The model under review builds one solid part; all positions refer to its coordinate system, in mm. Face numbers are marked on the shaded views. A direction names the side the tool comes from. Round coordinates to 2 decimals unless told otherwise and drop trailing zeros. Loops run counter-clockwise (first coordinate to the right, second up) from the corner with the lowest first, then second, coordinate; pieces in that order, holes last. Notation, with made-up numbers: (-25, 72.5) -> (-10, 72.5) arc R21 cw to (-10, 84.5) -> close; hole circle Ø5 at (80, 50.25). An arc over 180 degrees is marked (long way). Use a Markdown table: item, result. Add a question column.
1) Wall thickness on probe 1 along Z at (x, y) = (3, -4); probe 2 along Z at (x, y) = (7, -16.5); probe 3 along X at (y, z) = (-17.75, -14.75): over which ranges is each line inside the solid? List them lowest first.
2) Mouldability with a two-part tool opening along X and no side actions: class the marked faces 1, 2, 3 and 4 as released by +X, released by -X, zero draft, split by the parting line, or undercut.
3) Consider section A-A on y = -3.75. Give the boundary of the cut face in (x, z), plus the area to 3 significant figures.
4) Insertion check: pin 1 (2.5 mm diameter, centred on x = 11, z = -3, fed in from +Y). The pin has a flat end and moves straight along its axis. Give the tip position at first contact, or say it passes through.
5) For the marked faces 5, 6 and 7, list the 3-axis set-ups (+Z, -Z, +X, -X, +Y, -Y) from which the entire face can be reached by the end or side of a thin tool; tool diameter is ignored.
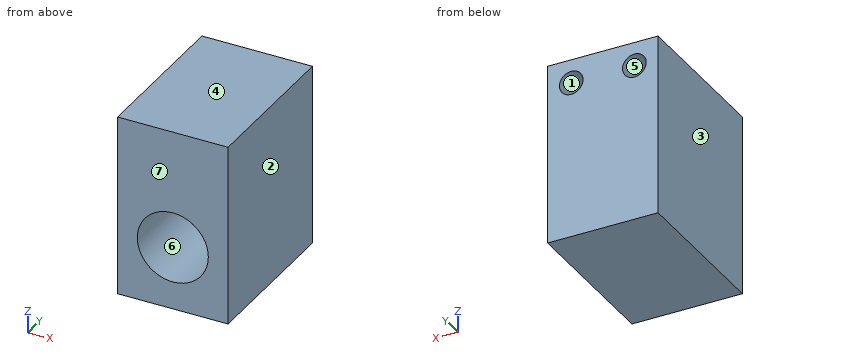
from build123d import *

# Parameters (mm, degrees)
SKETCH1_W                  = 14
SKETCH1_H                  = 23
BOSS_EXTRUDE1_DEPTH        = 20
F_3_0MM_DOWEL_HOLE1_D      = 3
F_3_0MM_DOWEL_HOLE1_DEPTH  = 5
F_3_0MM_DOWEL_HOLE1_TIP    = 0.901290929
M10X1_0_TAPPED_HOLE1_D     = 9
M10X1_0_TAPPED_HOLE1_DEPTH = 12
M10X1_0_TAPPED_HOLE1_TIP   = 2.703872786


with BuildPart() as part:
    # Sketch1 → Boss-Extrude1 (new body)
    with BuildSketch(Plane(origin=(0, 0, 0), x_dir=(1, 0, 0), z_dir=(0, 1, 0))):
        with Locations((7, 11.5)):
            Rectangle(SKETCH1_W, SKETCH1_H)
    extrude(amount=-BOSS_EXTRUDE1_DEPTH)

    # Ø3.0mm Dowel Hole1
    with Locations(Plane(origin=(0, 0, 0), x_dir=(1, 0, 0), z_dir=(0, 1, 0))):
        with Locations((3, 3), (11, 3)):
            Hole(F_3_0MM_DOWEL_HOLE1_D / 2, depth=F_3_0MM_DOWEL_HOLE1_DEPTH)
            with Locations((0, 0, -(F_3_0MM_DOWEL_HOLE1_DEPTH + F_3_0MM_DOWEL_HOLE1_TIP / 2))):  # 118° drill point
                Cone(0, F_3_0MM_DOWEL_HOLE1_D / 2, F_3_0MM_DOWEL_HOLE1_TIP, mode=Mode.SUBTRACT)

    # M10x1.0 Tapped Hole1
    with Locations(Plane(origin=(0, -20, 0), x_dir=(-1, 0, 0), z_dir=(0, -1, 0))):
        with Locations((-7, 15)):
            Hole(M10X1_0_TAPPED_HOLE1_D / 2, depth=M10X1_0_TAPPED_HOLE1_DEPTH)
            with Locations((0, 0, -(M10X1_0_TAPPED_HOLE1_DEPTH + M10X1_0_TAPPED_HOLE1_TIP / 2))):  # 118° drill point
                Cone(0, M10X1_0_TAPPED_HOLE1_D / 2, M10X1_0_TAPPED_HOLE1_TIP, mode=Mode.SUBTRACT)


solid = part.part
Result set:
| question | item | result |
|---|---|---|
| 1 | probe 1 | -23 to -4.5, -1.5 to 0 |
| 1 | probe 2 | -23 to -19.5, -10.5 to 0 |
| 1 | probe 3 | 0 to 2.51, 11.49 to 14 |
| 2 | face 1 | undercut |
| 2 | face 2 | released by +X |
| 2 | face 3 | released by -X |
| 2 | face 4 | zero draft |
| 3 | outline | (0, -23) -> (14, -23) -> (14, 0) -> (0, 0) -> close; hole circle Ø3 at (3, -3); hole circle Ø3 at (11, -3) |
| 3 | area | 308 mm2 |
| 4 | pin 1 | y = -5.15 |
| 5 | face 5 | +Y |
| 5 | face 6 | -Y |
| 5 | face 7 | +Z, -Z, +X, -X, -Y |
